from build123d import *

# Parameters (mm, degrees)
EXTRUDE_2_DEPTH     = 2.5
CUT_EXTRUDE_START   = 1
SKETCH_2_W          = 8
SKETCH_2_H          = 29
SKETCH_2_H_2        = 26
SKETCH_2_H_3        = 38
SKETCH_2_H_4        = 23
SKETCH_2_H_5        = 32
SKETCH_2_H_6        = 20
CUT_EXTRUDE_2_DEPTH = 1.5


with BuildPart() as part:
    # 草图3 → 凸台-拉伸2 (new body)
    with BuildSketch(Plane(origin=(0, 0, 0), x_dir=(1, 0, 0), z_dir=(0, 1, 0))):
        Polygon((90, 1), (-1, 1), (-1, -96), (72, -96), (72, -90), (90, -90), (90, -68), (72, -68), (72, -63), (90, -63), (90, -29), (72, -29), (36, -29), (36, -27), (72, -27), (72, -24), (90, -24), align=None)
    extrude(amount=EXTRUDE_2_DEPTH)

    # 草图2 → 切除-拉伸2 (cut)
    with BuildSketch(Plane(origin=(0, 0, 0), x_dir=(1, 0, 0), z_dir=(0, 1, 0)).offset(CUT_EXTRUDE_START)):
        with Locations((4, -14.5)):
            Rectangle(SKETCH_2_W, SKETCH_2_H)
        with Locations((13, -14.5)):
            Rectangle(SKETCH_2_W, SKETCH_2_H)
        with Locations((22, -14.5)):
            Rectangle(SKETCH_2_W, SKETCH_2_H)
        with Locations((31, -14.5)):
            Rectangle(SKETCH_2_W, SKETCH_2_H)
        with Locations((40, -13)):
            Rectangle(SKETCH_2_W, SKETCH_2_H_2)
        with Locations((4, -49)):
            Rectangle(SKETCH_2_W, SKETCH_2_H_3)
        with Locations((4, -82)):
            Rectangle(SKETCH_2_W, SKETCH_2_H_2)
        with Locations((49, -13)):
            Rectangle(SKETCH_2_W, SKETCH_2_H_2)
        with Locations((58, -13)):
            Rectangle(SKETCH_2_W, SKETCH_2_H_2)
        with Locations((67, -13)):
            Rectangle(SKETCH_2_W, SKETCH_2_H_2)
        with Locations((76, -11.5)):
            Rectangle(SKETCH_2_W, SKETCH_2_H_4)
        with Locations((85, -11.5)):
            Rectangle(SKETCH_2_W, SKETCH_2_H_4)
        with Locations((13, -49)):
            Rectangle(SKETCH_2_W, SKETCH_2_H_3)
        with Locations((22, -49)):
            Rectangle(SKETCH_2_W, SKETCH_2_H_3)
        with Locations((31, -49)):
            Rectangle(SKETCH_2_W, SKETCH_2_H_3)
        with Locations((40, -49)):
            Rectangle(SKETCH_2_W, SKETCH_2_H_3)
        with Locations((49, -49)):
            Rectangle(SKETCH_2_W, SKETCH_2_H_3)
        with Locations((58, -49)):
            Rectangle(SKETCH_2_W, SKETCH_2_H_3)
        with Locations((67, -49)):
            Rectangle(SKETCH_2_W, SKETCH_2_H_3)
        with Locations((76, -46)):
            Rectangle(SKETCH_2_W, SKETCH_2_H_5)
        with Locations((85, -46)):
            Rectangle(SKETCH_2_W, SKETCH_2_H_5)
        with Locations((13, -82)):
            Rectangle(SKETCH_2_W, SKETCH_2_H_2)
        with Locations((22, -82)):
            Rectangle(SKETCH_2_W, SKETCH_2_H_2)
        with Locations((31, -82)):
            Rectangle(SKETCH_2_W, SKETCH_2_H_2)
        with Locations((40, -82)):
            Rectangle(SKETCH_2_W, SKETCH_2_H_2)
        with Locations((49, -82)):
            Rectangle(SKETCH_2_W, SKETCH_2_H_2)
        with Locations((58, -82)):
            Rectangle(SKETCH_2_W, SKETCH_2_H_2)
        with Locations((67, -82)):
            Rectangle(SKETCH_2_W, SKETCH_2_H_2)
        with Locations((76, -79)):
            Rectangle(SKETCH_2_W, SKETCH_2_H_6)
        with Locations((85, -79)):
            Rectangle(SKETCH_2_W, SKETCH_2_H_6)
    extrude(amount=CUT_EXTRUDE_2_DEPTH, mode=Mode.SUBTRACT)


solid = part.part
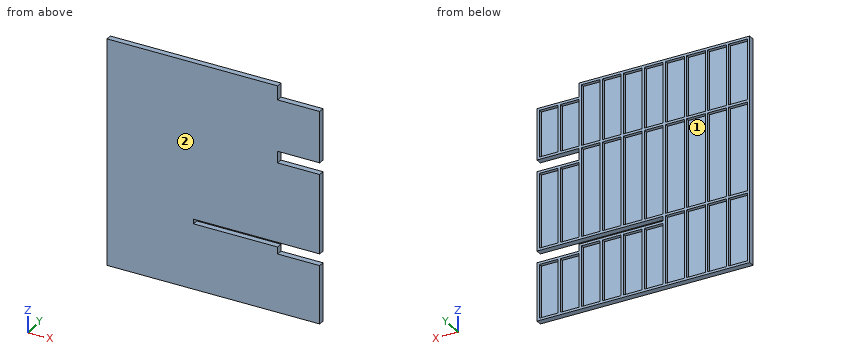
Can you work these out from the model? Positions are in its coordinate system, mm. Face numbers are marked on the shaded views. Coordinates: 2 decimals unless noted, no trailing zeros. Loops run counter-clockwise (first coordinate to the right, second up) from the corner with the lowest first, then second, coordinate; pieces in that order, holes last. Notation, with made-up numbers: (-18, 13.25) - (-9, 13.25) arc R23 cw to (-9, 39.25) - close; hole circle Ø3 at (15.25, -33.5). An arc over 180 degrees is marked (long way). Answer as a JSON object with one key per item and string values. Group by question number.
Item 1: If we section it at B-B (x = 6.5): List the corners of the cut face in (y, z) for me, plus the area to 3 significant figures.
Item 2: For pin 1 (6.5 mm diameter, centred on x = 67, z = 19.5, fed in from +Y); pin 2 (1.5 mm diameter, centred on x = 58.5, z = 25, fed in from -Y); pin 3 (1.2 mm diameter, centred on x = 79, y = 1.5, fed in from +Z), each with a flat end and sliding along its axis, tell me the tip position at first contact or that it passes through.
Item 3: If we section it at C-C (y = 1.55): State how many separate pieces and enclosed holes the cut face has, plus the area to 3 significant figures.
Item 4: If we section it at A-A (x = 55.5): List the corners of the cut face in (y, z) for me, plus the area to 4 significant figures.
Item 5: If we mould it in two halves opening along X, with no side actions, what happens to the marked faces 1 and 2? For each: released by +X, released by -X, zero draft, split by the parting line, or undercut.
Item 6: If I drill on L1, parallel to Z at x = 83.5, y = 2.15; L2, parallel to Z at x = 64.5, y = 2; L3, parallel to Z at x = 29, y = 1.9, over which ranges is the centre line in solid material (lowest first)? Write a range as from..to.
Returned:
{
 "1": {"outline": "(0, -1) - (2.5, -1) - (2.5, 0) - (1, 0) - (1, 29) - (2.5, 29) - (2.5, 30) - (1, 30) - (1, 68) - (2.5, 68) - (2.5, 69) - (1, 69) - (1, 95) - (2.5, 95) - (2.5, 96) - (0, 96) - close", "area": "103 mm²"},
 "2": {"pin 1": "stops at y = 1", "pin 2": "stops at y = 0", "pin 3": "stops at z = 90"},
 "3": {"separate pieces": "1", "enclosed holes": "30", "area": "1,410 mm²"},
 "4": {"outline": "(0, -1) - (2.5, -1) - (2.5, 0) - (1, 0) - (1, 26) - (2.5, 26) - (2.5, 27) - (0, 27) - close; (0, 29) - (2.5, 29) - (2.5, 30) - (1, 30) - (1, 68) - (2.5, 68) - (2.5, 69) - (1, 69) - (1, 95) - (2.5, 95) - (2.5, 96) - (0, 96) - close", "area": "102.5 mm²"},
 "5": {"face 1": "undercut", "face 2": "zero draft"},
 "6": {"L1": "z = -1..0, 23..24, 29..30, 62..63, 68..69, 89..90", "L2": "z = -1..0, 26..27, 29..30, 68..69, 95..96", "L3": "z = -1..0, 29..30, 68..69, 95..96"}
}
